Input: dimensioned drawing with shaded views. Units: mm. Origin: part minimum x, y, z. A direction names the side the tool comes from. Round coordinates to 2 decimals unless told otherwise and drop trailing zeros. Order: outer loops, then holes, each group sorted by start corner. A loop starts at its lowest first (then second) coordinate and runs counter-clockwise, first axis right, second up.
Item 1: Cut plane D-D on y = 312. Output: boundary loops of the cut face in (x, z), then the cut area to 3 significant figures.
Item 2: Cut plane B-B on z = 554.5. Output: boundary loops of the cut face in (x, y).
Item 3: First-contact query: pin 1 (12 mm diameter, centred on y = 291, z = 478, fed in from -X); pin 2 (12 mm diameter, centred on x = 335.5, y = 292, fed in from -Z); pin 3 (8 mm diameter, centred on x = 170.5, z = 277.5, fed in from +Y). Flat tips, straight axial feed; report the tip coordinate or a pass-through.
Item 4: Line query: L1, parallel to Z at x = 373.5, y = 436; L2, parallel to X at y = 370.5, z = 554; L3, parallel to Y at x = 432, z = 407. Output: solid intervals per line, ascending.
Item 5: Cut plane C-C on x = 310.5. Output: boundary loops of the cut face in (y, z), then the cut area to 3 significant figures.
Item 6: Cut plane A-A on y = 424. Output: boundary loops of the cut face in (x, z), then the cut area to 3 significant figures.
Item 7: Reachability of the marked faces 1 and 2 from +Z, -Z, +X, -X, +Y, -Y: full face, straight path, thin tool, end or side. Return the list, or none.
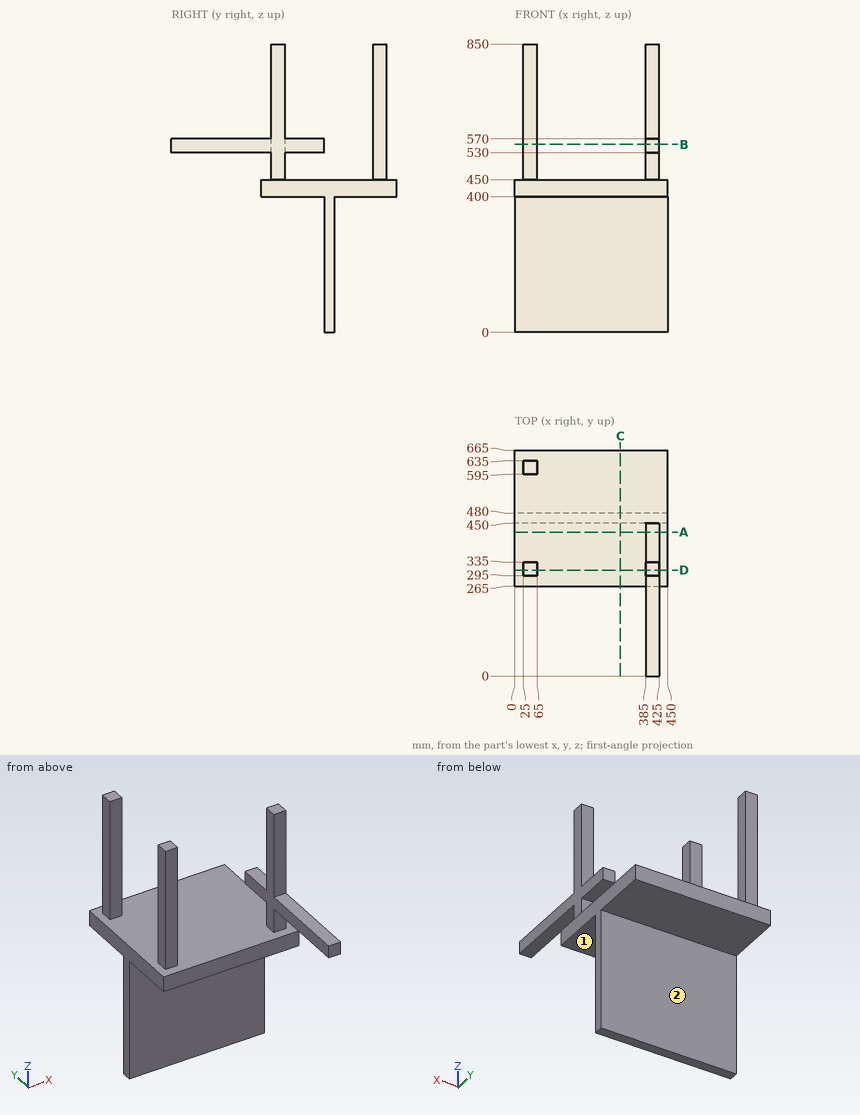
From the geometry:
1. outline: (0, 400) - (450, 400) - (450, 450) - (425, 450) - (425, 850) - (385, 850) - (385, 450) - (65, 450) - (65, 850) - (25, 850) - (25, 450) - (0, 450) - close
1. area: 54,500 mm2
2. outline: (25, 295) - (65, 295) - (65, 335) - (25, 335) - close; (25, 595) - (65, 595) - (65, 635) - (25, 635) - close; (385, 0) - (425, 0) - (425, 450) - (385, 450) - close
3. pin 1: stops at x = 25
3. pin 2: stops at z = 400
3. pin 3: stops at y = 480
4. L1: z = 400 to 450
4. L2: x = 385 to 425
4. L3: y = 265 to 665
5. outline: (265, 400) - (450, 400) - (450, 0) - (480, 0) - (480, 400) - (665, 400) - (665, 450) - (265, 450) - close
5. area: 32,000 mm2
6. outline: (0, 400) - (450, 400) - (450, 450) - (0, 450) - close; (385, 530) - (425, 530) - (425, 570) - (385, 570) - close
6. area: 24,100 mm2
7. face 1: -Z, +X, -X, -Y
7. face 2: -Z, +X, -X, +Y
